```python
from build123d import *

# Parameters (mm, degrees)
SKETCH1_W           = 107.763073452
SKETCH1_H           = 107.763073452
BOSS_EXTRUDE1_DEPTH = 3.175
CUT_EXTRUDE2_REACH  = 78.266
SKETCH4_R           = 8.5725
FILLET2_R           = 6.35
CUT_EXTRUDE3_REACH  = 78.266
SKETCH5_R           = 2.665000004
CUT_EXTRUDE4_REACH  = 78.266
SKETCH6_R           = 13.335


with BuildPart() as part:
    # Sketch1 → Boss-Extrude1 (new body)
    with BuildSketch(Plane.XY):
        Rectangle(SKETCH1_W, SKETCH1_H)
    extrude(amount=BOSS_EXTRUDE1_DEPTH)

    # Sketch4 → Cut-Extrude2 (cut, up to next)
    with BuildSketch(Plane.XY.offset(3.175), mode=Mode.PRIVATE) as cut_extrude2_sk1:
        Circle(SKETCH4_R)
    cut_extrude2_tool1 = extrude(cut_extrude2_sk1.sketch, amount=-CUT_EXTRUDE2_REACH, mode=Mode.PRIVATE) & part.part
    add(cut_extrude2_tool1.solids().sort_by_distance((0, 0, 3.175))[0], mode=Mode.SUBTRACT)

    # Fillet2
    fillet2_edges = [part.edges().sort_by_distance(p)[0] for p in [
        (-53.881536726, -53.881536726, 1.5875),
        (-53.881536726, 53.881536726, 1.5875),
        (53.881536726, 53.881536726, 1.5875),
        (53.881536726, -53.881536726, 1.5875),
    ]]
    fillet(fillet2_edges, radius=FILLET2_R)

    # Sketch5 → Cut-Extrude3 (cut, up to next)
    with BuildSketch(Plane(origin=(0, 0, 0), x_dir=(-1, 0, 0), z_dir=(0, 0, -1)), mode=Mode.PRIVATE) as cut_extrude3_sk1:
        with Locations((44.901280605, 44.901280605)):
            Circle(SKETCH5_R)
    cut_extrude3_tool1 = extrude(cut_extrude3_sk1.sketch, amount=-CUT_EXTRUDE3_REACH, mode=Mode.PRIVATE) & part.part
    # Sketch5 → Cut-Extrude3 (cut, up to next)
    with BuildSketch(Plane(origin=(0, 0, 0), x_dir=(-1, 0, 0), z_dir=(0, 0, -1)), mode=Mode.PRIVATE) as cut_extrude3_sk2:
        with Locations((44.901280605, -44.901280605)):
            Circle(SKETCH5_R)
    cut_extrude3_tool2 = extrude(cut_extrude3_sk2.sketch, amount=-CUT_EXTRUDE3_REACH, mode=Mode.PRIVATE) & part.part
    # Sketch5 → Cut-Extrude3 (cut, up to next)
    with BuildSketch(Plane(origin=(0, 0, 0), x_dir=(-1, 0, 0), z_dir=(0, 0, -1)), mode=Mode.PRIVATE) as cut_extrude3_sk3:
        with Locations((-44.901280605, -44.901280605)):
            Circle(SKETCH5_R)
    cut_extrude3_tool3 = extrude(cut_extrude3_sk3.sketch, amount=-CUT_EXTRUDE3_REACH, mode=Mode.PRIVATE) & part.part
    # Sketch5 → Cut-Extrude3 (cut, up to next)
    with BuildSketch(Plane(origin=(0, 0, 0), x_dir=(-1, 0, 0), z_dir=(0, 0, -1)), mode=Mode.PRIVATE) as cut_extrude3_sk4:
        with Locations((-44.901280605, 44.901280605)):
            Circle(SKETCH5_R)
    cut_extrude3_tool4 = extrude(cut_extrude3_sk4.sketch, amount=-CUT_EXTRUDE3_REACH, mode=Mode.PRIVATE) & part.part
    add(cut_extrude3_tool1.solids().sort_by_distance((-44.901281, 44.901281, 0))[0], mode=Mode.SUBTRACT)
    add(cut_extrude3_tool2.solids().sort_by_distance((-44.901281, -44.901281, 0))[0], mode=Mode.SUBTRACT)
    add(cut_extrude3_tool3.solids().sort_by_distance((44.901281, -44.901281, 0))[0], mode=Mode.SUBTRACT)
    add(cut_extrude3_tool4.solids().sort_by_distance((44.901281, 44.901281, 0))[0], mode=Mode.SUBTRACT)

    # Sketch6 → Cut-Extrude4 (cut, up to next)
    with BuildSketch(Plane.XY.offset(3.175), mode=Mode.PRIVATE) as cut_extrude4_sk1:
        with Locations((23.797678721, 23.797678721)):
            Circle(SKETCH6_R)
    cut_extrude4_tool1 = extrude(cut_extrude4_sk1.sketch, amount=-CUT_EXTRUDE4_REACH, mode=Mode.PRIVATE) & part.part
    # Sketch6 → Cut-Extrude4 (cut, up to next)
    with BuildSketch(Plane.XY.offset(3.175), mode=Mode.PRIVATE) as cut_extrude4_sk2:
        with Locations((-23.797678721, -23.797678721)):
            Circle(SKETCH6_R)
    cut_extrude4_tool2 = extrude(cut_extrude4_sk2.sketch, amount=-CUT_EXTRUDE4_REACH, mode=Mode.PRIVATE) & part.part
    add(cut_extrude4_tool1.solids().sort_by_distance((23.797679, 23.797679, 3.175))[0], mode=Mode.SUBTRACT)
    add(cut_extrude4_tool2.solids().sort_by_distance((-23.797679, -23.797679, 3.175))[0], mode=Mode.SUBTRACT)


solid = part.part
```
Read the model definition and answer for the solid it produces. Units are mm, in the model's axes. Coordinates: 2 decimals unless noted, no trailing zeros. Order: outer loops, then holes, each group sorted by start corner. A loop starts at its lowest first (then second) coordinate and runs counter-clockwise, first axis right, second up. Notation, with made-up numbers: (66.5, 11) - (88.5, 11) arc R13 ccw to (88.5, 27) - close; hole circle Ø9 at (-26, -34.5). An arc over 180 degrees is marked (long way). Answer as a JSON object with one key per item and string values. Group by question number.
Item 1: The mould has two halves that part along Y. Classify faces 1 (the face through (-42.24, -44.78, 1.57)), 2 (the face through (53.882, -1, 2)), 3 (the face through (-52.07, 51.97, 1.61)): +Y half, -Y half, draft (parallel to the pull), parting line (faces both ways), or undercut.
Item 2: Section A-A (x = 0) is taken. Give the vertices of the cut face in (y, z) (1 decimal).
Item 3: Section C-C (z = 0.8) is taken. State how many separate pieces and enclosed holes the cut face has, plus the area to 3 significant figures.
Item 4: A flat-ended cylindrical pin translates along its axis: P1, Ø4, axis at x = 36, y = 22, coming from the -Z side. Find the tip coordinate at first contact, or state that the pin passes through.
Item 5: Consider probe 1 along Y at (x, z) = (-48, 0.25); probe 2 along X at (y, z) = (-12, 2.1); probe 3 along X at (y, z) = (7, 2.3). Determine where each line is inside the solid, lowest interval first. Write a range as from..to.
Results are:
{
 "1": {"face 1": "undercut", "face 2": "draft", "face 3": "+Y half"},
 "2": {"outline": "(-53.9, 0) - (-8.6, 0) - (-8.6, 3.2) - (-53.9, 3.2) - close; (8.6, 0) - (53.9, 0) - (53.9, 3.2) - (8.6, 3.2) - close"},
 "3": {"separate pieces": "1", "enclosed holes": "7", "area": "10,100 mm^2"},
 "4": {"P1": "stops at z = 0"},
 "5": {"probe 1": "y = -53.86..53.86", "probe 2": "x = -53.88..-30.01, -17.58..53.88", "probe 3": "x = -53.88..-4.95, 4.95..53.88"}
}
